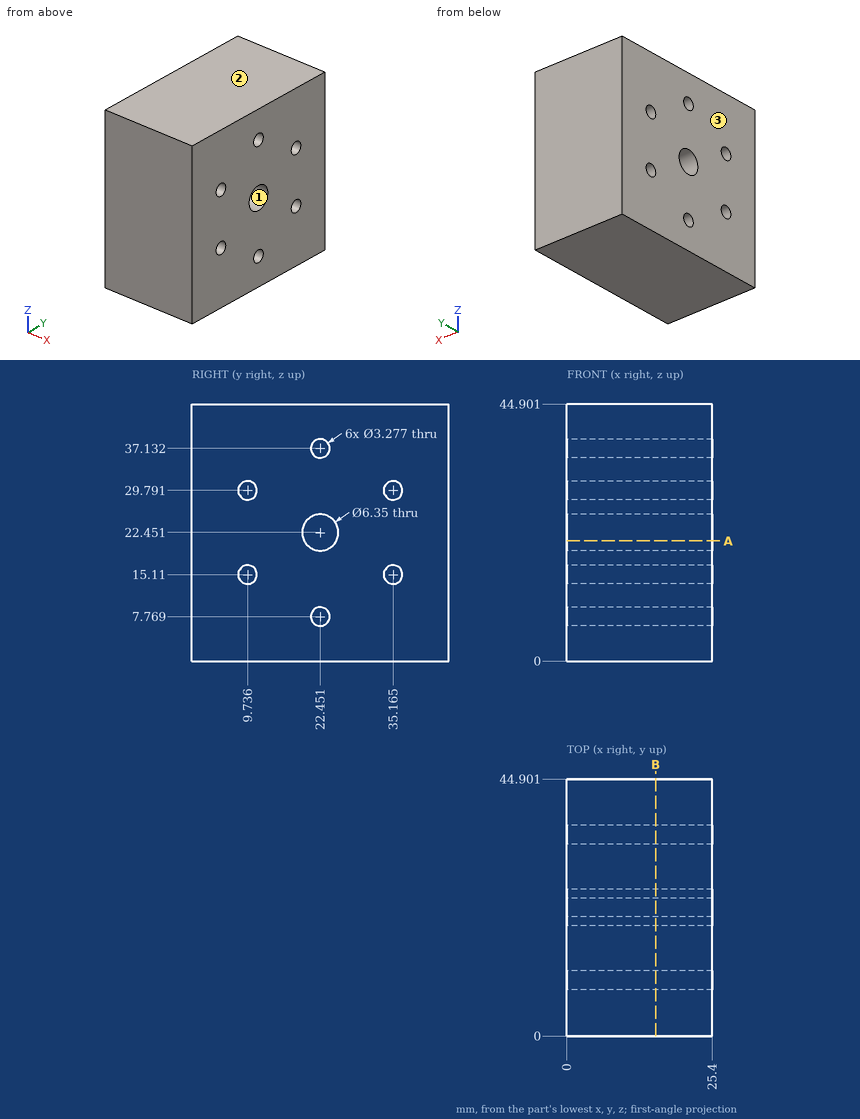
Geometry check sheet. Reference: drawing and pictorial views, mm from the part's lowest x, y, z. Coordinates: 2 decimals unless noted, no trailing zeros. Write each loop counter-clockwise with the first axis right and the second up, starting at its lowest first coordinate (ties: lowest second). Pieces come first, ordered by that corner, then holes. Notation, with made-up numbers: M -10.75,-13 L -4.75,-13 A10 ccw -4.75,1 Z; hole C -24.75,82.5 d2. An arc over 180 degrees is marked long. Use one line per item in the form item = value.
Item 1: Release check for a two-part mould opening along Z. For the marked faces 1, 2 and 3 record: pulls with the +Z half, pulls with the -Z half, needs draft (parallel to the pull), parting line crosses it, or undercut.
Answer below:
face_1 = undercut
face_2 = pulls with the +Z half
face_3 = needs draft
Item 2: Sectioned sample at A-A, the plane z = 21. Record the cut outline in (x, y) (1 decimal).
Answer below:
outline = M 0,0 L 25.4,0 L 25.4,19.6 L 0,19.6 Z; M 0,25.3 L 25.4,25.3 L 25.4,44.9 L 0,44.9 Z
Item 3: Sectioned sample at B-B, the plane x = 15.5. State how many separate pieces and enclosed holes the cut face has, and give its area (3 significant figures).
Answer below:
separate_pieces = 1
enclosed_holes = 7
area = 1,930 mm^2
Item 4: Material ranges on L1, parallel to Z at x = 8.25, y = 35; L2, parallel to Z at x = 6, y = 36; L3, parallel to Y at x = 19, z = 21 (1 decimal), recorded low to high. Write a range as from..to.
Answer below:
L1 = 0..13.48, 16.74..28.16, 31.42..44.9
L2 = 0..13.7, 16.52..28.38, 31.2..44.9
L3 = 0..19.6, 25.3..44.9
